Autodesk Inventor part; units mm, degrees
ref_plane "YZ Plane" through (0, 0, 0) normal (1, 0, 0) x (0, 1, 0)
ref_plane "XZ Plane" through (0, 0, 0) normal (0, 1, 0) x (-1, 0, 0)
ref_plane "XY Plane" through (0, 0, 0) normal (0, 0, 1) x (1, 0, 0)
sketch "Sketch1" plane through (0, 0, 0) normal (0, 0, 1) x (1, 0, 0)
  line L0 (0, 0) -> (286, 0)
  line L1 (286, 0) -> (286, 40)
  line L2 (286, 40) -> (0, 40)
  line L3 (0, 40) -> (0, 0)
  dimension "d0" = 286
  dimension "d1" = 40
extrude "Extrusion1" add sketch "Sketch1" along normal blind 5
sketch "Sketch2" plane through (0, 0, 5) normal (0, 0, 1) x (1, 0, 0)
  line L0 (286, 40) -> (0, 40)
  line L1 (0, 0) -> (286, 0)
  line L2 (0, 40) -> (0, 0)
  point P0 (43, 30)
  point P1 (43, 10)
  dimension "d4" = 10
  dimension "d6" = 43
  dimension "d40" = 20
  dimension "d41" = 10
hole "Hole1" at (43, 30, 5) at (43, 10, 5) direction (0, 0, -1) diameter 4.5 end through all
pattern_linear "Rectangular Pattern1" count 5 spacing 50 along (1, 0, 0) of "Hole1"
sketch "Sketch3" plane through (0, 0, 5) normal (0, 0, 1) x (1, 0, 0)
  line L0 (286, 40) -> (0, 40)
  line L1 (0, 40) -> (0, 0)
  line L2 (286, 0) -> (286, 40)
  point P0 (68.3759, 20)
  point P1 (217.6241, 5)
  dimension "d17" = 150
  dimension "d18" = 20
  dimension "d19" = 15
  dimension "d20" = 68.3759
  dimension "d21" = 68.3759
hole "Hole2" at (68.3759, 20, 5) at (217.6241, 5, 5) direction (0, 0, -1) diameter 4.5 end through all
sketch "Sketch4" plane through (0, 0, 5) normal (0, 0, 1) x (1, 0, 0)
  line L0 (286, 40) -> (0, 40)
  line L1 (0, 0) -> (286, 0)
  line L2 (0, 40) -> (0, 0)
  line L3 (286, 0) -> (286, 40)
  point P0 (12.5, 32.5)
  point P1 (12.5, 7.5)
  point P2 (273.5, 32.5)
  point P3 (273.5, 7.5)
  dimension "d29" = 7.5
  dimension "d30" = 7.5
  dimension "d31" = 12.5
  dimension "d32" = 12.5
hole "Hole3" at (12.5, 32.5, 5) at (12.5, 7.5, 5) at (273.5, 32.5, 5) at (273.5, 7.5, 5) direction (0, 0, -1) diameter 4.5 end through all
sketch "Sketch5" plane through (0, 0, 5) normal (0, 0, 1) x (1, 0, 0)
  line L0 (286, 40) -> (0, 40)
  line L1 (0, 40) -> (0, 0)
  line L2 (286, 0) -> (286, 40)
  point P0 (25, 35)
  point P1 (261, 35)
  dimension "d42" = 5
  dimension "d43" = 25
  dimension "d44" = 25
hole "Hole4" at (25, 35, 5) at (261, 35, 5) direction (0, 0, -1) diameter 3 end through all
properties part number "Top_Slider Piece 1" material "Wood (Oak)"
For this review, take the finished solid that the model builds, in its own axes (mm). Give positions to 0.01 mm unless a question says otherwise; leave off trailing zeros. One line per question, with ' | ' between items.
1) The part is to be moulded in two halves that separate along Y. For faces 1 (the flat face through (141, 0, 2)), 2 (the flat face through (286, 20, 2)), 3 (the cylindrical face through (95.196, 10.488, 2.465)), 4 (the cylindrical face through (271.27, 32.79, 2.46)), say which applies: +Y half, -Y half, draft (parallel to the pull), parting line (faces both ways), or undercut.
Resolved:
face 1: -Y half | face 2: draft | face 3: undercut | face 4: undercut
2) To check wall thickness, follow probe 1 along Y at (x, z) = (143, 3.2); probe 2 along X at (y, z) = (10.5, 1.25); probe 3 along X at (y, z) = (32.5, 2.45). State the ranges of each line that lie inside material, in increasing order.
Resolved:
probe 1: y = 0 to 7.75, 12.25 to 27.75, 32.25 to 40 | probe 2: x = 0 to 40.81, 45.19 to 90.81, 95.19 to 140.81, 145.19 to 190.81, 195.19 to 240.81, 245.19 to 286 | probe 3: x = 0 to 10.25, 14.75 to 271.25, 275.75 to 286
3) We need section A-A (z = 3.4). Give the number of separate pieces and of enclosed holes in the cut face, plus the area to 3 significant figures.
Resolved:
separate pieces: 1 | enclosed holes: 18 | area: 11,200 mm2
